from build123d import *

# Parameters (mm, degrees)
SKETCH1_R           = 5
SKETCH1_R_2         = 2
BOSS_EXTRUDE1_DEPTH = 2
BOSS_EXTRUDE2_DEPTH = 48
BOSS_EXTRUDE3_DEPTH = 1
CUT_EXTRUDE2_DEPTH  = 36
BOSS_EXTRUDE4_DEPTH = 21
BOSS_EXTRUDE5_DEPTH = 1
SKETCH8_W           = 4
SKETCH8_H           = 15.623627573
BOSS_EXTRUDE6_DEPTH = 9
SKETCH11_R          = 5
SKETCH11_R_2        = 2.5
BOSS_EXTRUDE7_DEPTH = 5


with BuildPart() as part:
    # Sketch1 → Boss-Extrude1 (new body)
    with BuildSketch(Plane.XY):
        with BuildLine():
            Line((-12.5, 0), (12.5, 0))
            Line((12.5, 0), (9.876921901, 16.564101584))
            ThreePointArc((9.876921901, 16.564101584), (0, 25), (-9.876921901, 16.564101584))
            Line((-9.876921901, 16.564101584), (-12.5, 0))
        make_face()
        with Locations((0, 12.5)):
            Circle(SKETCH1_R, mode=Mode.SUBTRACT)
        with Locations((5, 6.1)):
            Circle(SKETCH1_R_2, mode=Mode.SUBTRACT)
        with Locations((-5, 6.1)):
            Circle(SKETCH1_R_2, mode=Mode.SUBTRACT)
        with Locations((0, 21)):
            Circle(SKETCH1_R_2, mode=Mode.SUBTRACT)
    extrude(amount=BOSS_EXTRUDE1_DEPTH)

    # Sketch2 → Boss-Extrude2 (add)
    with BuildSketch(Plane(origin=(0, 0, 50), x_dir=(-1, 0, 0), z_dir=(0, 0, -1))):
        Polygon((12.5, 0), (-12.5, 0), (-11.866563146, 4), (11.866563146, 4), align=None)
    extrude(amount=BOSS_EXTRUDE2_DEPTH)

    # Sketch3 → Boss-Extrude3 (add, symmetric)
    with BuildSketch(Plane.XY.offset(22)):
        with BuildLine():
            ThreePointArc((5.92615314, 15.93846095), (0, 21), (-5.92615314, 15.93846095))
            Line((-5.92615314, 15.93846095), (-7.183281573, 8))
            Line((-7.183281573, 8), (-7.816718427, 4))
            Line((-7.816718427, 4), (7.816718427, 4))
            Line((7.816718427, 4), (7.183281573, 8))
            Line((7.183281573, 8), (5.92615314, 15.93846095))
        make_face()
        with BuildLine():
            Line((5.92615314, 15.93846095), (5.098508377, 21.164836764))
            ThreePointArc((5.098508377, 21.164836764), (0, 23), (-5.098508377, 21.164836764))
            Line((-5.098508377, 21.164836764), (-5.92615314, 15.93846095))
            ThreePointArc((-5.92615314, 15.93846095), (0, 21), (5.92615314, 15.93846095))
        make_face()
    extrude(amount=BOSS_EXTRUDE3_DEPTH, both=True)

    # Sketch4 → Cut-Extrude2 (cut)
    with BuildSketch(Plane(origin=(0, 4, 0), x_dir=(1, 0, 0), z_dir=(0, 1, 0))):
        with BuildLine():
            Line((-12.5, -22), (-4.423680321, -37.330461847))
            ThreePointArc((-4.423680321, -37.330461847), (0, -40), (4.423680321, -37.330461847))
            Line((4.423680321, -37.330461847), (12.5, -22))
            Line((12.5, -22), (16.181982352, -22))
            Line((16.181982352, -22), (16.181982352, -36.988467345))
            Line((16.181982352, -36.988467345), (30.820243312, -58.391823719))
            Line((30.820243312, -58.391823719), (-16.187396411, -58.391823719))
            Line((-16.187396411, -58.391823719), (-16.187396411, -22))
            Line((-16.187396411, -22), (-12.5, -22))
        make_face()
    extrude(amount=-CUT_EXTRUDE2_DEPTH, mode=Mode.SUBTRACT)

    # Sketch6 → Boss-Extrude4 (add)
    with BuildSketch(Plane.XY.offset(2)):
        Polygon((-7.866563146, 4), (-7.816718427, 4), (-5.827077182, 16.564101584), (-9.876921901, 16.564101584), (-11.866563146, 4), align=None)
        Polygon((7.866563146, 4), (11.866563146, 4), (9.876921901, 16.564101584), (5.827077182, 16.564101584), (7.816718427, 4), align=None)
    extrude(amount=BOSS_EXTRUDE4_DEPTH)

    # Sketch7 → Boss-Extrude5 (add, symmetric)
    with BuildSketch(Plane.XY.offset(33)):
        with BuildLine():
            ThreePointArc((3.823881283, 19.623627573), (2.032022953, 20.645430251), (0, 21))
            Line((0, 21), (0, 4))
            Line((0, 4), (5.827077182, 4))
            Line((5.827077182, 4), (3.823881283, 19.623627573))
        make_face()
        with BuildLine():
            ThreePointArc((0, 21), (-2.032022953, 20.645430251), (-3.823881283, 19.623627573))
            Line((-3.823881283, 19.623627573), (-5.827077182, 4))
            Line((-5.827077182, 4), (0, 4))
            Line((0, 4), (0, 21))
        make_face()
    extrude(amount=BOSS_EXTRUDE5_DEPTH, both=True)

    # Sketch8 → Boss-Extrude6 (add)
    with BuildSketch(Plane(origin=(0, 0, 32), x_dir=(-1, 0, 0), z_dir=(0, 0, -1))):
        with Locations((0.057647427, 11.811813787)):
            Rectangle(SKETCH8_W, SKETCH8_H)
    extrude(amount=BOSS_EXTRUDE6_DEPTH)

    # Sketch11 → Boss-Extrude7 (add)
    with BuildSketch(Plane.XZ):
        with Locations(Location((0, 10, 0), (0, 0, 90))):
            Circle(SKETCH11_R)
        with Locations(Location((0, 10, 0), (0, 0, 270))):
            Circle(SKETCH11_R_2, mode=Mode.SUBTRACT)
    extrude(amount=BOSS_EXTRUDE7_DEPTH)


solid = part.part
Here's how the part is built. I have some questions about the finished solid (model axes, mm). A direction names the side the tool comes from. Coordinates: 2 decimals unless noted, no trailing zeros. Order: outer loops, then holes, each group sorted by start corner. A loop starts at its lowest first (then second) coordinate and runs counter-clockwise, first axis right, second up.
Item 1: If we section it at B-B on y = 6.1: List the corners of the cut face in (x, z) for me.
Result sheet:
outline: (-11.53, 0) - (-7, 0) - (-7, 2) - (-7.48, 2) - (-7.48, 21) - (7.48, 21) - (7.48, 2) - (7, 2) - (7, 0) - (11.53, 0) - (11.53, 23) - (1.94, 23) - (1.94, 32) - (5.56, 32) - (5.56, 34) - (-5.56, 34) - (-5.56, 32) - (-2.06, 32) - (-2.06, 23) - (-11.53, 23) - close; (-3, 0) - (3, 0) - (3, 2) - (-3, 2) - close
Item 2: For faces 4 (the face through (0, 13, 34)), 5 (the face through (2, 19, 2)), 6 (the face through (-2.5, 4, 29.7)), 7 (the face through (0, 0, 10)), which set-ups out of +Z, -Z, +X, -X, +Y, -Y let a thin tool reach every point of the face, with its end or its side?
Result sheet:
face 4: +Z, +X, -X, +Y
face 5: none
face 6: +Y
face 7: -Y
Item 3: If we section it at C-C on z = 10: List the corners of the cut face in (x, y) for me.
Result sheet:
outline: (-12.5, 0) - (-5, 0) - (-5, -5) - (-2.5, -5) - (-2.5, 0) - (2.5, 0) - (2.5, -5) - (5, -5) - (5, 0) - (12.5, 0) - (9.88, 16.56) - (5.83, 16.56) - (7.82, 4) - (-7.82, 4) - (-5.83, 16.56) - (-9.88, 16.56) - close
Item 4: If we section it at A-A on x = 0: State how many separate pieces and enclosed holes the cut face has, plus the area to 3 significant figures.
Result sheet:
separate pieces: 3
enclosed holes: 0
area: 412 mm2
Item 5: For P1, Ø5, axis at y = 9, z = 19, coming from the +X side; P2, Ø12, axis at x = -5.5, y = 17.5, coming from the +Z side; P3, Ø1.5, axis at x = -1, z = 9.5, coming from the -Y side, each with a flat end and sliding along its axis, tell me the tip position at first contact or that it passes through.
Result sheet:
P1: stops at x = 11.47
P2: stops at z = 34
P3: stops at y = 0
Item 6: If we mould it in two halves opening along Z, with no side actions, what happens to faces 1 (the face through (-5.458, 18.897, 22.014)), 2 (the face through (0, 14, 21)), 3 (the face through (0, 2, 40))? For each: +Z half, -Z half, draft (parallel to the pull), parting line (faces both ways), or undercut.
Result sheet:
face 1: draft
face 2: undercut
face 3: +Z half
Item 7: If we section it at D-D on y = -1.5: List the corners of the cut face in (x, z) for me.
Result sheet:
outline: circle Ø10 at (0, 10); hole circle Ø5 at (0, 10)
Item 8: I need wall thicknesses on line 1 (Y direction, x = 0, z = 1); line 2 (Z direction, x = -2, y = 20); line 3 (Z direction, x = -3, y = 12.5). Which ranges of each line are inside material? Lowest first, please.
Result sheet:
line 1: y = 0 to 7.5, 17.5 to 19, 23 to 25
line 2: z = 0 to 2, 21 to 23, 32 to 34
line 3: z = 21 to 23, 32 to 34
